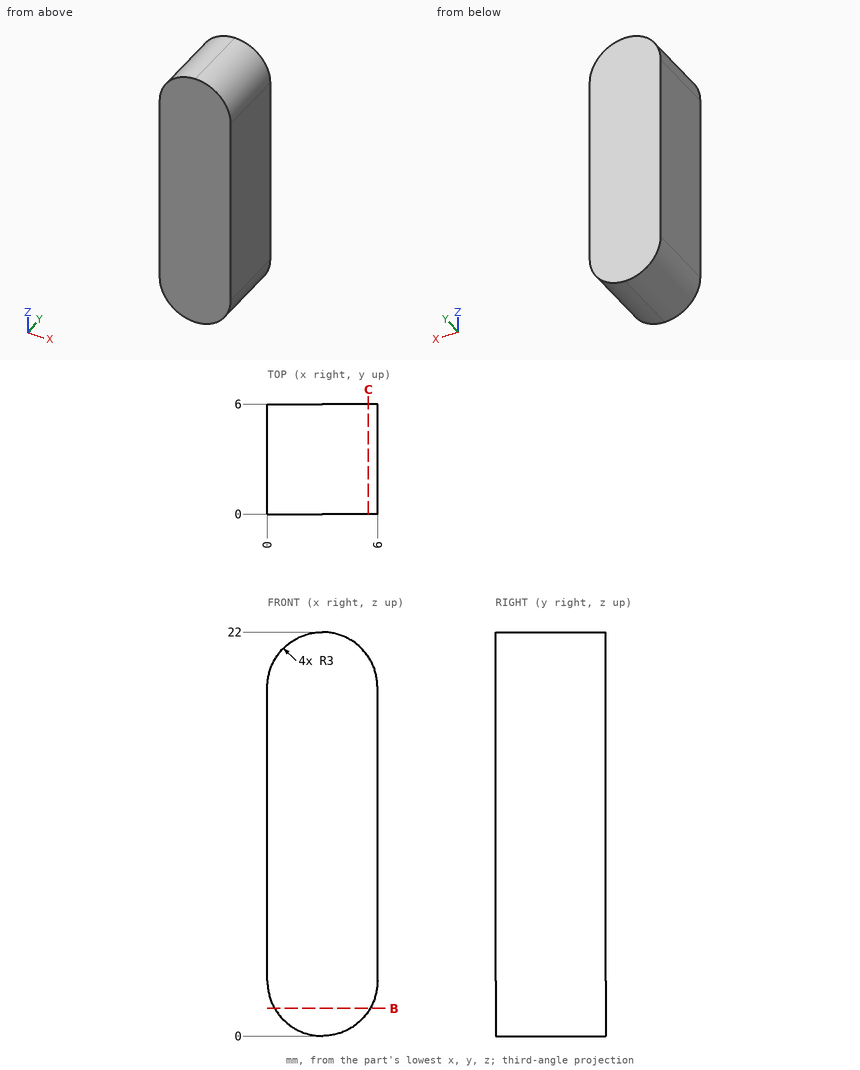
Drawing for the job (mm, zero at the part's lowest x, y, z). Round coordinates to 2 decimals unless told otherwise and drop trailing zeros. Order: outer loops, then holes, each group sorted by start corner. A loop starts at its lowest first (then second) coordinate and runs counter-clockwise, first axis right, second up. Notation, with made-up numbers: (28.25, 43) -> (79.25, 43) arc R18 ccw to (79.25, 49) -> close; hole circle Ø6 at (63, -17). An arc over 180 degrees is marked (long way). Write item = value, one per line. Start each with the question number.
(1) Pin check, flat tip, straight feed: P1, Ø1.5, axis at x = 5, y = 1.5, coming from the -Z side. Stop position of the tip, or through.
(2) Cut at B-B, the plane z = 1.5. List the corners of the cut face in (x, y), then the cut area to 3 significant figures.
(3) Cut at C-C, the plane x = 5.5. List the corners of the cut face in (y, z), then the cut area to 3 significant figures.
(4) Probe line 1 (Z direction, x = 2, y = 1.1); line 2 (X direction, y = 1.4, z = 2); line 3 (X direction, y = 5.3, z = 19.5). List the from-to ranges inside material, lowest first. Write a range as [from, to].
Model answer:
q1.P1 = 0.27
q2.outline = (0.4, 0) -> (5.6, 0) -> (5.6, 6) -> (0.4, 6) -> close
q2.area = 31.2 mm2
q3.outline = (0, 1.34) -> (6, 1.34) -> (6, 20.66) -> (0, 20.66) -> close
q3.area = 116 mm2
q4.line_1 = [0.17, 21.83]
q4.line_2 = [0.17, 5.83]
q4.line_3 = [0.04, 5.96]
